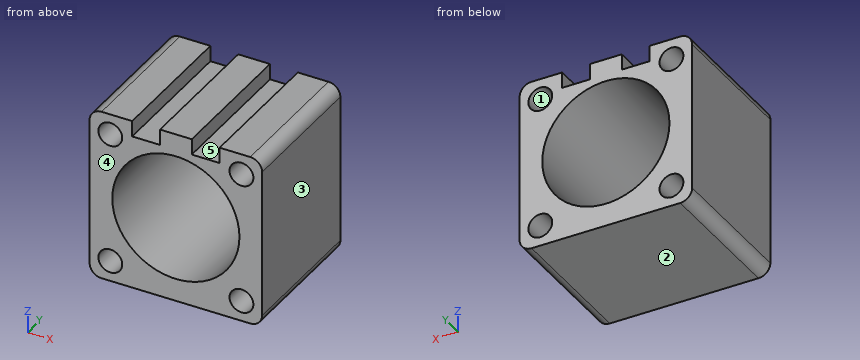
from build123d import *

# Parameters (mm, degrees)
F0_W     = 43.4
F0_H     = 43.4
F0_R     = 3
F0_R_2   = 16
F1_DEPTH = 17.5
F2_W     = 7
F2_H     = 35
F3_DEPTH = 4
F4_R     = 3


with BuildPart() as f1:
    # F0 (on Front) → F1 (new body, symmetric)
    with BuildSketch(Plane.XZ):
        Rectangle(F0_W, F0_H)
        with Locations((-16.5, -16.5)):
            Circle(F0_R, mode=Mode.SUBTRACT)
        with Locations((16.5, -16.5)):
            Circle(F0_R, mode=Mode.SUBTRACT)
        with Locations((-16.5, 16.5)):
            Circle(F0_R, mode=Mode.SUBTRACT)
        Circle(F0_R_2, mode=Mode.SUBTRACT)
        with Locations((16.5, 16.5)):
            Circle(F0_R, mode=Mode.SUBTRACT)
    extrude(amount=F1_DEPTH, both=True)

    # F2 (on face) → F3 (cut)
    with BuildSketch(Plane.XY.offset(21.7)):
        with Locations((-7.5, 0)):
            Rectangle(F2_W, F2_H)
        with Locations((7.5, 0)):
            Rectangle(F2_W, F2_H)
    extrude(amount=-F3_DEPTH, mode=Mode.SUBTRACT)

    # F4
    f4_edges = [f1.edges().sort_by_distance(p)[0] for p in [
        (-21.7, 0, 21.7),
        (21.7, 0, 21.7),
        (21.7, 0, -21.7),
        (-21.7, 0, -21.7),
    ]]
    fillet(f4_edges, radius=F4_R)


solid = f1.part
Part model, mm, in its own coordinate system. Face numbers are marked on the shaded views. A direction names the side the tool comes from. Coordinates: 2 decimals unless noted, no trailing zeros. Loops run counter-clockwise (first coordinate to the right, second up) from the corner with the lowest first, then second, coordinate; pieces in that order, holes last. Notation, with made-up numbers: M 39.5,9.5 L 48.5,9.5 A26 cw 48.5,26.5 Z; hole C 77,69 d3. An arc over 180 degrees is marked long. Use a Markdown table: item, result. Add a question column.
Q1. Which spindle directions (+Z, -Z, +X, -X, +Y, -Y) get a long thin tool onto all of the face, cutting with end or side? Do the marked faces 4 and 5. Say none if no direction does.
Q2. Probe L1, parallel to Z at x = -16.5, y = 3.5; L2, parallel to Z at x = 0, y = -5; L3, parallel to X at y = 1.5, z = 14.5. List the from-to ranges inside material, lowest first.
Q3. Cut at C-C (x = 0). Write the cut outline in (y, z), and give its area (3 significant figures).
Q4. Cut at B-B (x = 8). Write the cut outline in (y, z).
Q5. Mould opens along X. For the marked faces 1, 2 and 3 say: +X half, -X half, draft (parallel to the pull), parting line (faces both ways), or undercut.
Q6. Pin check, flat tips, straight feed: P1, Ø5.5, axis at x = -16.5, z = 16.5, coming from the -Y side (3 decimals); P2, Ø1.5, axis at x = -9, y = -2.5, coming from the +Z side. Stop position of each tip, or through.
Q7. Cut at A-A (y = 7). Write the cut outline in (x, z), and give its area (3 significant figures).
Worked out:
| question | item | result |
|---|---|---|
| 1 | face 4 | +Z, -Z, +X, -X, -Y |
| 1 | face 5 | +Z, +Y, -Y |
| 2 | L1 | z = -21.7 to -19.5, -13.5 to 13.5, 19.5 to 21.7 |
| 2 | L2 | z = -21.7 to -16, 16 to 21.7 |
| 2 | L3 | x = -21.7 to -18.74, -14.26 to -6.76, 6.76 to 14.26, 18.74 to 21.7 |
| 3 | outline | M -17.5,-21.7 L 17.5,-21.7 L 17.5,-16 L -17.5,-16 Z; M -17.5,16 L 17.5,16 L 17.5,21.7 L -17.5,21.7 Z |
| 3 | area | 399 mm2 |
| 4 | outline | M -17.5,-21.7 L 17.5,-21.7 L 17.5,-13.86 L -17.5,-13.86 Z; M -17.5,13.86 L 17.5,13.86 L 17.5,17.7 L -17.5,17.7 Z |
| 5 | face 1 | undercut |
| 5 | face 2 | draft |
| 5 | face 3 | +X half |
| 6 | P1 | passes through |
| 6 | P2 | stops at z = 17.7 |
| 7 | outline | M -21.7,-18.7 A3 ccw -18.7,-21.7 L 18.7,-21.7 A3 ccw 21.7,-18.7 L 21.7,18.7 A3 ccw 18.7,21.7 L 11,21.7 L 11,17.7 L 4,17.7 L 4,21.7 L -4,21.7 L -4,17.7 L -11,17.7 L -11,21.7 L -18.7,21.7 A3 ccw -21.7,18.7 Z; hole C -16.5,-16.5 d6; hole C -16.5,16.5 d6; hole C 0,0 d32; hole C 16.5,-16.5 d6; hole C 16.5,16.5 d6 |
| 7 | area | 902 mm2 |
